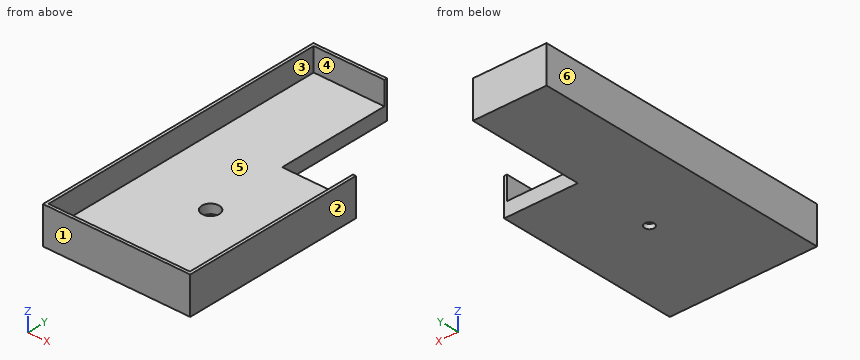
from build123d import *

# Parameters (mm, degrees)
F1_DEPTH = 6
F2_W     = 1.25
F2_H     = 126.5
F2_H_2   = 1.25
F2_H_3   = 77.75
F3_DEPTH = 10
F4_R     = 3.75
F5_DEPTH = 4
F6_R     = 2.1
F7_DEPTH = 2


with BuildPart() as f1:
    # F0 (on Top) → F1 (new body)
    with BuildSketch(Plane.XY):
        Polygon((-31.5, -64.5), (31.5, -64.5), (31.5, 14.5), (0, 14.5), (0, 64.5), (-31.5, 64.5), align=None)
    extrude(amount=F1_DEPTH)

    # F2 (on face) → F3 (join)
    with BuildSketch(Plane.XY.offset(6)):
        Polygon((0, 64.5), (-31.5, 64.5), (-31.5, 63.25), (-30.25, 63.25), (-29, 63.25), (0, 63.25), align=None)
        with Locations((-30.875, 0)):
            Rectangle(F2_W, F2_H)
        with Locations((-30.875, -63.875)):
            Rectangle(F2_W, F2_H_2)
        Polygon((30.25, -63.25), (-30.25, -63.25), (-30.25, -64.5), (31.5, -64.5), (31.5, -63.25), align=None)
        with Locations((30.875, -24.375)):
            Rectangle(F2_W, F2_H_3)
    extrude(amount=F3_DEPTH)

    # F4 (on face) → F5 (cut)
    with BuildSketch(Plane.XY.offset(6)):
        with Locations((0, -19.654689)):
            Circle(F4_R)
    extrude(amount=-F5_DEPTH, mode=Mode.SUBTRACT)

    # F6 (on face) → F7 (cut, through all)
    with BuildSketch(Plane.XY.offset(2)):
        with Locations((0, -19.654689)):
            Circle(F6_R)
    extrude(amount=-F7_DEPTH, mode=Mode.SUBTRACT)


solid = f1.part
Source: CAD feature listing. Evaluate the final solid. Frame: model axes, mm. Face numbers are marked on the shaded views. A direction names the side the tool comes from. Round coordinates to 2 decimals unless told otherwise and drop trailing zeros. Loops run counter-clockwise (first coordinate to the right, second up) from the corner with the lowest first, then second, coordinate; pieces in that order, holes last.
Q1. Section B-B, the plane x = -19. Return loops of the section in (y, z).
Q2. Section C-C, the plane y = 4.5. Return loops of the section in (x, z).
Q3. Ray query, line 1 (X direction, y = -18.5, z = 8.75); line 2 (Y direction, x = -1, z = 9); line 3 (Y direction, x = 5, z = 9.5). Return the intervals inside material, ascending.
Q4. Section A-A, the plane z = 14. Return loops of the section in (x, y).
Q5. Section D-D, the plane x = 11.5. Return loops of the section in (y, z), plus the area to 4 significant figures.
Q6. Mould query, pull axis Y, two halves, no side actions, for the marked faces 1, 2 and 3. Classes: pulls with the +Y half, pulls with the -Y half, needs draft (parallel to the pull), parting line crosses it, or undercut.
Q7. Access query for the marked faces 4, 5 and 6. Directions: +Z, -Z, +X, -X, +Y, -Y. A direction counts if a zero-diameter tool reaches every point of the face in a straight line with its end or side. Return the directions, or none.
Q8. First-contact query: P1, Ø18, axis at x = 8.5, y = -19, coming from the +Z side; P2, Ø6, axis at x = 25, z = 11.5, coming from the +Y side; P3, Ø7, axis at x = 0, y = -19.65, coming from the +Z side. Flat tips, straight axial feed; report the tip coordinate or a pass-through.
Solutions:
1. outline: (-64.5, 0) - (64.5, 0) - (64.5, 16) - (63.25, 16) - (63.25, 6) - (-63.25, 6) - (-63.25, 16) - (-64.5, 16) - close
2. outline: (-31.5, 0) - (31.5, 0) - (31.5, 16) - (30.25, 16) - (30.25, 6) - (-30.25, 6) - (-30.25, 16) - (-31.5, 16) - close
3. line 1: x = -31.5 to -30.25, 30.25 to 31.5
3. line 2: y = -64.5 to -63.25, 63.25 to 64.5
3. line 3: y = -64.5 to -63.25
4. outline: (-31.5, -64.5) - (31.5, -64.5) - (31.5, 14.5) - (30.25, 14.5) - (30.25, -63.25) - (-30.25, -63.25) - (-30.25, 63.25) - (0, 63.25) - (0, 64.5) - (-31.5, 64.5) - close
5. outline: (-64.5, 0) - (14.5, 0) - (14.5, 6) - (-63.25, 6) - (-63.25, 16) - (-64.5, 16) - close
5. area: 486.5 mm2
6. face 1: pulls with the -Y half
6. face 2: needs draft
6. face 3: undercut
7. face 4: +Z, +X
7. face 5: +Z
7. face 6: +Z, -Z, -X, +Y, -Y
8. P1: stops at z = 6
8. P2: stops at y = -63.25
8. P3: stops at z = 2
